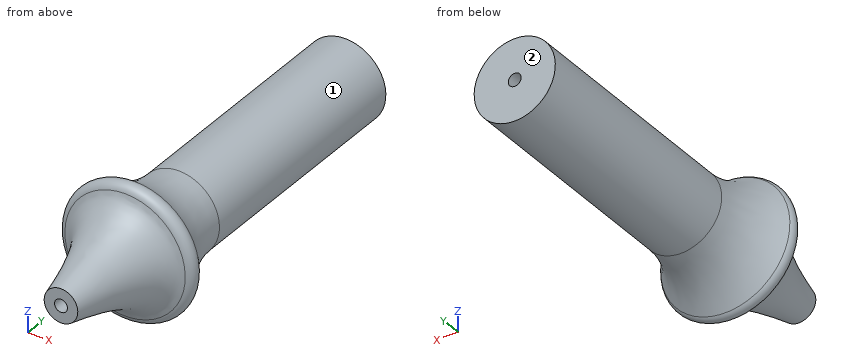
```python
from build123d import *


with BuildPart() as part:
    # Sketch2 → Revolve1 (revolve)
    with BuildSketch(Plane(origin=(0, 0, 0), x_dir=(0, 0, -1), z_dir=(1, 0, 0))):
        with BuildLine():
            Line((-10, 79.984026871), (-10, 20))
            ThreePointArc((-10, 20), (-11.529300925, 11.508521396), (-15.925023202, 4.084129443))
            ThreePointArc((-15.925023202, 4.084129443), (-16.348258147, 2.040451452), (-14.8325, 0.6058))
            add(Edge.make_bspline(
                [(-14.8325, 0.6058), (-14.786589527, 0.594107912), (-14.720151881, 0.577188139), (-14.636942478, 0.555651214), (-14.584628983, 0.541606051), (-14.538694782, 0.529056302), (-14.496115893, 0.516807178), (-14.455377323, 0.504752713), (-14.415703886, 0.492601586), (-14.376608725, 0.480213978), (-14.337823066, 0.467258765), (-14.299073296, 0.453804959), (-14.260077477, 0.439967714), (-14.220832936, 0.425142489), (-14.181003545, 0.409828499), (-14.140639226, 0.39342794), (-14.099539827, 0.376264866), (-14.057643188, 0.358051468), (-14.015003626, 0.338576095), (-13.971270318, 0.318244004), (-13.926716478, 0.296334648), (-13.88091734, 0.273357564), (-13.834012449, 0.248879897), (-13.785997304, 0.222646856), (-13.736545511, 0.195147367), (-13.685880417, 0.165637059), (-13.63383256, 0.134329981), (-13.580202235, 0.101238986), (-13.525196985, 0.065829097), (-13.468489978, 0.028394376), (-13.410218497, -0.011527982), (-13.350168278, -0.053791023), (-13.288470654, -0.098900311), (-13.224788811, -0.146603335), (-13.159241207, -0.197326808), (-13.091855296, -0.251341181), (-13.022233522, -0.308401649), (-12.950733187, -0.369268693), (-12.87684498, -0.433607317), (-12.800942833, -0.50216692), (-12.722558879, -0.574690204), (-12.64180647, -0.651653184), (-12.558631713, -0.733330072), (-12.473007863, -0.820056033), (-12.384606656, -0.911877967), (-12.293655943, -1.009413525), (-12.19993662, -1.112809578), (-12.103181234, -1.222292158), (-12.003658589, -1.33855085), (-11.901000777, -1.461694366), (-11.795279131, -1.592272191), (-11.686428516, -1.730738869), (-11.574152693, -1.877409894), (-11.458536394, -2.032929305), (-11.339441079, -2.197751566), (-11.216906306, -2.372586938), (-11.090456233, -2.557718159), (-10.960339372, -2.754078467), (-10.826403135, -2.962267921), (-10.688322214, -3.182881678), (-10.546388799, -3.416882377), (-10.399982006, -3.664853532), (-10.249381335, -3.927893894), (-10.094533615, -4.206969526), (-9.93478729, -4.502781144), (-9.770600526, -4.816720029), (-9.601692365, -5.149846675), (-9.427661931, -5.50326599), (-9.248775965, -5.878475674), (-9.064645901, -6.276835238), (-8.87533319, -6.699902872), (-8.680516638, -7.149341121), (-8.480119182, -7.626897717), (-8.27419422, -8.134593345), (-8.062173697, -8.674341942), (-7.844473046, -9.248617697), (-7.620378546, -9.859652358), (-7.390143634, -10.510239162), (-7.15351637, -11.203263925), (-6.91022293, -11.941816272), (-6.660409366, -12.729407317), (-6.403463868, -13.569619022), (-6.13955877, -14.466660747), (-5.86859751, -15.425045871), (-5.58995818, -16.449575), (-5.30410545, -17.54587051), (-5.010246169, -18.719716622), (-4.708679684, -19.977884286), (-4.417462856, -21.247043384), (-4.229902291, -22.098318051), (-4.143040834, -22.5)],
                knots=[0, 0, 0, 0, 0.0026864, 0.003887524, 0.004873731, 0.005757813, 0.006587588, 0.007385986, 0.008166831, 0.008940344, 0.009711391, 0.010485479, 0.011266269, 0.012057584, 0.012864206, 0.013685875, 0.014528001, 0.015389717, 0.016276196, 0.017186037, 0.018124349, 0.019091365, 0.020091502, 0.021124214, 0.022193786, 0.02329991, 0.024448714, 0.025637823, 0.026873089, 0.028157979, 0.029490658, 0.030878236, 0.032321667, 0.033824319, 0.035389905, 0.037021117, 0.038721252, 0.040494021, 0.042345363, 0.044276569, 0.046293536, 0.048400508, 0.050601853, 0.052903384, 0.055310916, 0.057829088, 0.060465162, 0.063223709, 0.066113781, 0.069142731, 0.072314292, 0.075640292, 0.079129636, 0.082787821, 0.086628416, 0.090659818, 0.094893736, 0.099340772, 0.104016433, 0.108930498, 0.114098239, 0.119534774, 0.125258904, 0.131284732, 0.137631752, 0.144321681, 0.151373222, 0.158810235, 0.166659266, 0.174942777, 0.183694449, 0.192940456, 0.202718271, 0.21306062, 0.224006047, 0.235599981, 0.247884808, 0.260909978, 0.274731834, 0.289408721, 0.305001629, 0.321583099, 0.339229092, 0.358021891, 0.378056499, 0.39943301, 0.422263423, 0.446671009, 0.472795467, 0.496098755, 0.496098755, 0.496098755, 0.496098755], degree=3))
            Line((-4.143040834, -22.5), (-1.5875, -22.5))
            Line((-1.5875, -22.5), (-1.5875, 79.984026871))
            Line((-1.5875, 79.984026871), (-10, 79.984026871))
        make_face()
    revolve(axis=Axis((0, -48.8258, 0), (0, 1, 0)))


solid = part.part
```
Build history of the part. All positions in model axes, mm. Face numbers are marked on the shaded views. A direction names the side the tool comes from. Give positions to 0.01 mm unless a question says otherwise; leave off trailing zeros. Loops run counter-clockwise (first coordinate to the right, second up) from the corner with the lowest first, then second, coordinate; pieces in that order, holes last.
Item 1: Which spindle directions (+Z, -Z, +X, -X, +Y, -Y) get a long thin tool onto all of the face, cutting with end or side? Do the marked faces 1 and 2. Say none if no direction does.
Answers follow:
face 1: +Y
face 2: +Z, -Z, +X, -X, +Y
Item 2: Flat gauge pins, fed straight in: pin 1 (10 mm diameter, centred on y = 65.5, z = 2.5, fed in from +X); pin 2 (5 mm diameter, centred on x = -2, z = 11, fed in from -Y); pin 3 (1.5 mm diameter, centred on y = 43.5, z = 3.5, fed in from +X); pin 4 (3.5 mm diameter, centred on x = 0, z = 0, fed in from +Y). Where does each tip first touch, or does it go through?
Answers follow:
pin 1: stops at x = 10
pin 2: stops at y = -7.15
pin 3: stops at x = 9.61
pin 4: stops at y = 79.98
Item 3: Slice it at A-A, the plane y = 40. List the corners of the cut face in (x, z) (1 decimal).
Answers follow:
outline: circle Ø20 at (0, 0); hole circle Ø3.2 at (0, 0)
Item 4: Drill centre lines: line 1 (X direction, y = 30.5, z = 0); line 2 (X direction, y = 15, z = 0); line 3 (Y direction, x = 12, z = -9.5). Where is each one in solid material? Low to high.
Answers follow:
line 1: x = -10 to -1.59, 1.59 to 10
line 2: x = -10.52 to -1.59, 1.59 to 10.52
line 3: y = 0.79 to 4.83
Item 5: Slice it at B-B, the plane y = 7.5. List the corners of the cut face in (x, z) (1 decimal), and give its area (3 significant figures).
Answers follow:
outline: circle Ø26.9 at (0, 0); hole circle Ø3.2 at (0, 0)
area: 561 mm2
